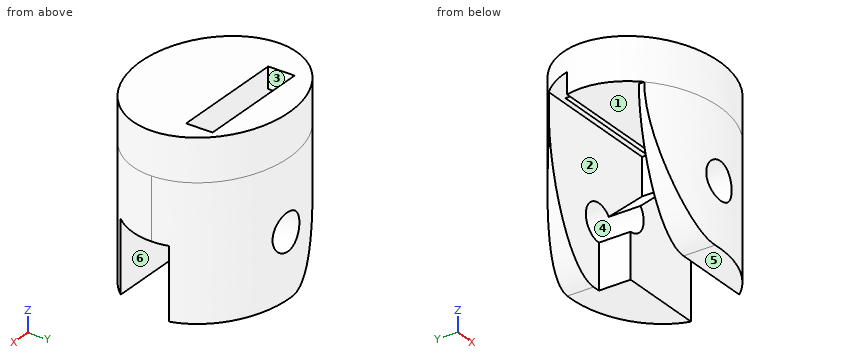
```python
from build123d import *

# Parameters (mm, degrees)
SKETCH1_RX          = 8.5
SKETCH1_RY          = 7
BOSS_EXTRUDE1_DEPTH = 4
SKETCH5_RX          = 8.5
SKETCH5_RY          = 7
BOSS_EXTRUDE2_DEPTH = 12.5
SKETCH6_R           = 1.75
CUT_EXTRUDE1_DEPTH  = 20
SKETCH8_W           = 17
SKETCH8_H           = 5.5
CUT_EXTRUDE4_DEPTH  = 6.7
SKETCH9_W           = 11
SKETCH9_H           = 2.5
CUT_EXTRUDE5_DEPTH  = 5.5
CUT_EXTRUDE7_DEPTH  = 5.5
CUT_EXTRUDE8_DEPTH  = 3
SCALE1_SCALE        = 2


with BuildPart() as part:
    # Sketch1 → Boss-Extrude1 (new body)
    with BuildSketch(Plane.XY):
        with Locations(Location((0, 0), (0, 0, 0))):
            Ellipse(SKETCH1_RX, SKETCH1_RY)
    extrude(amount=BOSS_EXTRUDE1_DEPTH)

    # Sketch5 → Boss-Extrude2 (add)
    with BuildSketch(Plane(origin=(0, 0, 0), x_dir=(-1, 0, 0), z_dir=(0, 0, -1))):
        with Locations(Location((0, 0), (0, 0, -180))):
            Ellipse(SKETCH5_RX, SKETCH5_RY)
    extrude(amount=BOSS_EXTRUDE2_DEPTH)

    # Sketch6 → Cut-Extrude1 (cut)
    with BuildSketch(Plane(origin=(0, 10, 0), x_dir=(1, 0, 0), z_dir=(0, 1, 0))):
        with Locations(Location((0.2, 6.5, 0), (0, 0, 270))):
            Circle(SKETCH6_R)
        with BuildLine():
            Line((-8.5, 12.5), (-8.5, 0))
            Line((-8.5, 0), (-6.5, 0))
            add(Edge.make_bspline(
                [(-6.5, 0), (-6.5, 5.077021549), (-3.853880334, 12.5), (-0.5, 12.5)],
                knots=[0, 0, 0, 0, 1, 1, 1, 1], degree=3))
            Line((-0.5, 12.5), (-8.5, 12.5))
        make_face()
    extrude(amount=-CUT_EXTRUDE1_DEPTH, mode=Mode.SUBTRACT)

    # Sketch8 → Cut-Extrude4 (cut)
    with BuildSketch(Plane.XY.offset(-12.5)):
        with Locations((0, -1.25)):
            Rectangle(SKETCH8_W, SKETCH8_H)
    extrude(amount=CUT_EXTRUDE4_DEPTH, mode=Mode.SUBTRACT)

    # Sketch9 → Cut-Extrude5 (cut)
    with BuildSketch(Plane.XY.offset(4)):
        with Locations((0.5, 2.75)):
            Rectangle(SKETCH9_W, SKETCH9_H)
    extrude(amount=-CUT_EXTRUDE5_DEPTH, mode=Mode.SUBTRACT)

    # Sketch10 → Cut-Extrude7 (cut)
    with BuildSketch(Plane(origin=(0, -4, 0), x_dir=(1, 0, 0), z_dir=(0, 1, 0))):
        Polygon((-8.5, 0), (3.5, 0), (5.725540357, 5.8), (-8.5, 5.8), align=None)
    extrude(amount=CUT_EXTRUDE7_DEPTH, mode=Mode.SUBTRACT)

    # Sketch11 → Cut-Extrude8 (cut)
    with BuildSketch(Plane(origin=(0, 1.5, 0), x_dir=(-1, 0, 0), z_dir=(0, -1, 0))):
        Polygon((-0.2, 6.5), (-0.2, 12.5), (8.5, 12.5), (8.5, 1.5), (8.5, -2), (-6, -2), (-6, 1.5), align=None)
    extrude(amount=-CUT_EXTRUDE8_DEPTH, mode=Mode.SUBTRACT)


with BuildPart() as part_1:
    # Scale1: scaled about (1.259390776, -0.158043462, -2.5785604)
    add(part.part.scale(SCALE1_SCALE).moved(Location((-1.259390776, 0.158043462, 2.5785604))))


solid = part_1.part
```
Could you check a few things on this model? Use its own coordinates, in mm. Face numbers are marked on the shaded views. A direction names the side the tool comes from. Round coordinates to 2 decimals unless told otherwise and drop trailing zeros. Answer as CSV lines item,"result".
1. On a 3-axis mill with a long thin cutter (end or side, diameter ignored), from which of +Z, -Z, +X, -X, +Y, -Y can I reach the whole of each face in a straight line? I mean the marked faces 1, 2 and 3. Say none if no direction works.
Filled in:
face 1,"-Z, -X"
face 2,"-X"
face 3,"+Z, -Z"
2. We'd pull the mould along Z, two halves only. Please class the marked faces 4, 5 and 6: +Z half, -Z half, draft (parallel to the pull), parting line (faces both ways), or undercut.
Filled in:
face 4,"undercut"
face 5,"-Z half"
face 6,"draft"
3. I want a section at A-A on x = 0.5. Count the separate pieces of the cut face and the enclosed holes in it, then the cut area to 3 significant figures.
Filled in:
separate pieces,"4"
enclosed holes,"0"
area,"433 mm^2"
4. For pin 1 Ø7.5 at (x, z) = (1.5, -10.5) entering from -Y; pin 2 Ø6 at (x, z) = (4, 2.5) entering from +Y; pin 3 Ø8 at (x, z) = (4.5, -10.5) entering from -Y, each with a flat end and sliding along its axis, tell me the tip position at first contact or that it passes through.
Filled in:
pin 1,"stops at y = -13.81"
pin 2,"stops at y = 14.03"
pin 3,"stops at y = -13.67"
